Model file for the job. Use its own axes, mm. A direction names the side the tool comes from. Round coordinates to 2 decimals unless told otherwise and drop trailing zeros. Order: outer loops, then holes, each group sorted by start corner. A loop starts at its lowest first (then second) coordinate and runs counter-clockwise, first axis right, second up. Notation, with made-up numbers: M 5,-15.5 L 48,-15.5 A21 cw 48,22.5 Z; hole C 7,-30.75 d8. An arc over 180 degrees is marked long. Return JSON: item names as keys, results as strings. Group by question number.
Item 1: Which spindle directions (+Z, -Z, +X, -X, +Y, -Y) get a long thin tool onto all of the face, cutting with end or side? Do faces 1 (the face through (10, 0, 44.45)), 2 (the face through (0, -22.225, 4)), 3 (the face through (0, 25.4, 4)). Say none if no direction does.
Item 2: Slice it at A-A on y = 18. Write the cut outline in (x, z) (3 decimals), then the cut area to 3 significant figures.
Item 3: Probe line 1 along X through (y, z) = (0, -182) (3 decimals); line 2 along Y through (x, z) = (-8.25, 43) (3 decimals); line 3 along Z through (x, y) = (10, 11). List the from-to ranges inside material, lowest first.
Item 4: Slice it at C-C on x = 4.5. Write the cut outline in (y, z) (3 decimals).
Item 5: Pin check, flat tips, straight feed: pin 1 Ø6.5 at (x, y) = (3.5, 5.5) entering from -Z; pin 2 Ø3.5 at (y, z) = (-24.5, 47) entering from +X. Stop position of each tip, or through.
Item 6: Slice it at B-B on z = 192. Write the cut outline in (x, y) (3 decimals), then the cut area to 3 significant figures.
Item 7: Pull direction X, two halves, no side cores. Call faces 4 (the face through (9.525, 0, -150)), 5 (the face through (9.525, 0, 153)), 6 (the face through (-10, -2, -252.476)), 7 (the face through (12.7, 0, 153)): pulls with the +X half, pulls with the -X half, needs draft (parallel to the pull), parting line crosses it, or undercut.
from build123d import *

# Parameters (mm, degrees)
SKETCH1_W           = 25.4
SKETCH1_H           = 50.8
SKETCH1_W_2         = 19.05
SKETCH1_H_2         = 44.45
BOSS_EXTRUDE1_DEPTH = 252.476
SKETCH2_W           = 6.35
SKETCH2_H           = 50.8
CUT_EXTRUDE1_DEPTH  = 12.7


with BuildPart() as part:
    # Sketch1 → Boss-Extrude1 (new, symmetric)
    with BuildSketch(Plane.XY):
        Rectangle(SKETCH1_W, SKETCH1_H)
        Rectangle(SKETCH1_W_2, SKETCH1_H_2, mode=Mode.SUBTRACT)
    extrude(amount=BOSS_EXTRUDE1_DEPTH, both=True)

    # Sketch2 → Cut-Extrude1 (cut)
    with BuildSketch(Plane(origin=(12.7, 0, 0), x_dir=(0, 0, -1), z_dir=(1, 0, 0))):
        with Locations((47.625, 0)):
            Rectangle(SKETCH2_W, SKETCH2_H)
        with Locations((-47.625, 0)):
            Rectangle(SKETCH2_W, SKETCH2_H)
    extrude(amount=-CUT_EXTRUDE1_DEPTH, mode=Mode.SUBTRACT)


solid = part.part
Output values:
{
 "1": {"face 1": "+X, +Y, -Y", "face 2": "+Z, -Z", "face 3": "+Z, -Z, +X, -X, +Y"},
 "2": {"outline": "M -12.7,-252.476 L -9.525,-252.476 L -9.525,252.476 L -12.7,252.476 Z; M 9.525,-252.476 L 12.7,-252.476 L 12.7,-50.8 L 9.525,-50.8 Z; M 9.525,-44.45 L 12.7,-44.45 L 12.7,44.45 L 9.525,44.45 Z; M 9.525,50.8 L 12.7,50.8 L 12.7,252.476 L 9.525,252.476 Z", "area": "3,170 mm²"},
 "3": {"line 1": "-12.7 to -9.525, 9.525 to 12.7", "line 2": "-25.4 to -22.225, 22.225 to 25.4", "line 3": "-252.48 to -50.8, -44.45 to 44.45, 50.8 to 252.48"},
 "4": {"outline": "M -25.4,-252.476 L -22.225,-252.476 L -22.225,-50.8 L -25.4,-50.8 Z; M -25.4,-44.45 L -22.225,-44.45 L -22.225,44.45 L -25.4,44.45 Z; M -25.4,50.8 L -22.225,50.8 L -22.225,252.476 L -25.4,252.476 Z; M 22.225,-252.476 L 25.4,-252.476 L 25.4,-50.8 L 22.225,-50.8 Z; M 22.225,-44.45 L 25.4,-44.45 L 25.4,44.45 L 22.225,44.45 Z; M 22.225,50.8 L 25.4,50.8 L 25.4,252.476 L 22.225,252.476 Z"},
 "5": {"pin 1": "through", "pin 2": "x = 0"},
 "6": {"outline": "M -12.7,-25.4 L 12.7,-25.4 L 12.7,25.4 L -12.7,25.4 Z; hole M -9.525,-22.225 L 9.525,-22.225 L 9.525,22.225 L -9.525,22.225 Z", "area": "444 mm²"},
 "7": {"face 4": "undercut", "face 5": "undercut", "face 6": "needs draft", "face 7": "pulls with the +X half"}
}
